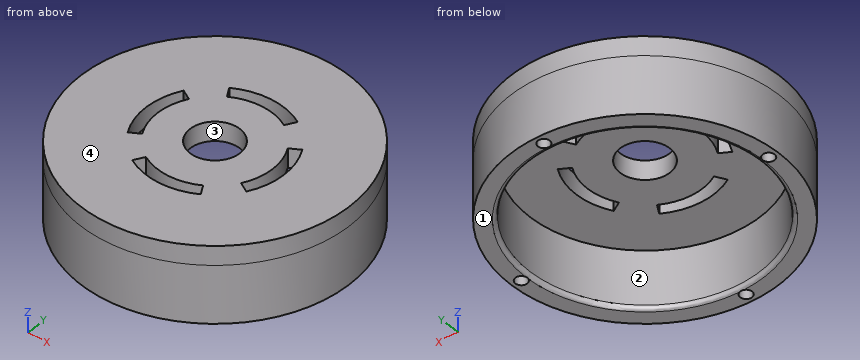
from build123d import *

# Parameters (mm, degrees)
SKETCH_2_R          = 35
SKETCH_2_R_2        = 6.5
EXTRUDE_1_DEPTH     = 5
EXTRUDE_START       = 15
SKETCH_3_R          = 35
SKETCH_3_R_2        = 30.05
EXTRUDE_2_DEPTH     = 15
SKETCH_4_R          = 1.55
CUT_EXTRUDE_1_DEPTH = 10
FILLET_1_R          = 1
CUT_EXTRUDE_2_DEPTH = 52.720402193


with BuildPart() as part:
    # 草图2 → 凸台-拉伸1 (new body)
    with BuildSketch(Plane.XY):
        Circle(SKETCH_2_R)
        Circle(SKETCH_2_R_2, mode=Mode.SUBTRACT)
    extrude(amount=EXTRUDE_1_DEPTH)

    # 草图3 → 凸台-拉伸2 (add)
    with BuildSketch(Plane(origin=(0, 0, 0), x_dir=(-1, 0, 0), z_dir=(0, 0, -1)).offset(EXTRUDE_START)):
        Circle(SKETCH_3_R)
        Circle(SKETCH_3_R_2, mode=Mode.SUBTRACT)
    extrude(amount=-EXTRUDE_2_DEPTH)

    # 草图4 → 切除-拉伸1 (cut)
    with BuildSketch(Plane(origin=(0, 0, -15), x_dir=(-1, 0, 0), z_dir=(0, 0, -1))):
        with Locations((0, 32.5)):
            Circle(SKETCH_4_R)
        with Locations((32.5, 0)):
            Circle(SKETCH_4_R)
        with Locations((0, -32.5)):
            Circle(SKETCH_4_R)
        with Locations((-32.5, 0)):
            Circle(SKETCH_4_R)
    extrude(amount=-CUT_EXTRUDE_1_DEPTH, mode=Mode.SUBTRACT)

    # 圆角1
    # the kernel refuses this fillet: 1 mm, written as the material it takes off along each edge
    with BuildSketch(Plane(origin=(0, 0, -15), x_dir=(-1, 0, 0), z_dir=(0, -1, 0))) as fillet_1_piece_1:
        with BuildLine():
            CenterArc((30.05 + FILLET_1_R, -FILLET_1_R), FILLET_1_R, 90, 90)
            Line((30.05, -FILLET_1_R), (30.05, 0))
            Line((30.05, 0), (30.05 + FILLET_1_R, 0))
        make_face()
    revolve(axis=Axis((0, 0, -15), (0, 0, -1)), mode=Mode.SUBTRACT)

    # 草图5 → 切除-拉伸2 (cut, through all)
    with BuildSketch(Plane(origin=(0, 0, 0), x_dir=(-1, 0, 0), z_dir=(0, 0, -1))):
        with BuildLine():
            Line((12.990381057, -7.5), (15.588457268, -9))
            ThreePointArc((15.588457268, -9), (18, 0), (15.588457268, 9))
            Line((15.588457268, 9), (12.990381057, 7.5))
            ThreePointArc((12.990381057, 7.5), (15, 0), (12.990381057, -7.5))
        make_face()
        with BuildLine():
            Line((-7.5, 12.990381057), (-9, 15.588457268))
            ThreePointArc((-9, 15.588457268), (0, 18), (9, 15.588457268))
            Line((9, 15.588457268), (7.5, 12.990381057))
            ThreePointArc((7.5, 12.990381057), (0, 15), (-7.5, 12.990381057))
        make_face()
        with BuildLine():
            Line((-7.5, -12.990381057), (-9, -15.588457268))
            ThreePointArc((-9, -15.588457268), (0, -18), (9, -15.588457268))
            Line((9, -15.588457268), (7.5, -12.990381057))
            ThreePointArc((7.5, -12.990381057), (0, -15), (-7.5, -12.990381057))
        make_face()
        with BuildLine():
            Line((-12.990381057, 7.5), (-15.588457268, 9))
            ThreePointArc((-15.588457268, 9), (-18, 0), (-15.588457268, -9))
            Line((-15.588457268, -9), (-12.990381057, -7.5))
            ThreePointArc((-12.990381057, -7.5), (-15, 0), (-12.990381057, 7.5))
        make_face()
    extrude(amount=-CUT_EXTRUDE_2_DEPTH, mode=Mode.SUBTRACT)


solid = part.part
Could you check a few things on this model? Use its own coordinates, in mm. Face numbers are marked on the shaded views. A direction names the side the tool comes from. Round coordinates to 2 decimals unless told otherwise and drop trailing zeros. Order: outer loops, then holes, each group sorted by start corner. A loop starts at its lowest first (then second) coordinate and runs counter-clockwise, first axis right, second up.
Q1. Imagine slicing it at C-C, the plane y = -14. State how many separate pieces and enclosed holes the cut face has, then the cut area to 3 significant figures.
Geometry says:
separate pieces: 3
enclosed holes: 0
area: 458 mm2
Q2. Imagine slicing it at A-A, the plane x = 32.5. List the corners of the cut face in (y, z) for me.
Geometry says:
outline: (-12.99, -15) - (-1.55, -15) - (-1.55, -5) - (1.55, -5) - (1.55, -15) - (12.99, -15) - (12.99, 5) - (-12.99, 5) - close
Q3. Which directions (+Z, -Z, +X, -X, +Y, -Y) give clear straight access to the entire face, cutting with the end or side of a thin tool? Please do the marked faces 1 and 2.
Geometry says:
face 1: -Z, +X, -X, +Y, -Y
face 2: -Z
Q4. I'm going to push flat-ended pins straight in: P1, Ø1.9, axis at x = 0, y = -32.5, coming from the -Z side; P2, Ø2, axis at x = 19.5, z = -5.5, coming from the -Y side; P3, Ø3, axis at x = -24.5, z = -3.5, coming from the -Y side. Where does each tip first touch, or does it pass through?
Geometry says:
P1: stops at z = -5
P2: stops at y = -29.71
P3: stops at y = -26.38
Q5. Thinking about a two-plate mould opening in Y: for the marked faces 3 and 4, which applies, released by +Y, released by -Y, zero draft, split by the parting line, or undercut?
Geometry says:
face 3: undercut
face 4: zero draft
Q6. Please list where these lines run through material, in increasing order: probe 1 along Y at (x, z) = (0, 2.45); probe 2 along X at (y, z) = (32.5, -11.25); probe 3 along Y at (x, z) = (0, -9.75).
Geometry says:
probe 1: y = -35 to -18, -15 to -6.5, 6.5 to 15, 18 to 35
probe 2: x = -12.99 to -1.55, 1.55 to 12.99
probe 3: y = -35 to -34.05, -30.95 to -30.05, 30.05 to 30.95, 34.05 to 35
